Source: CAD feature listing. Evaluate the final solid. Frame: model axes, mm. Face numbers are marked on the shaded views. A direction names the side the tool comes from. Give positions to 0.01 mm unless a question says otherwise; leave off trailing zeros. Order: outer loops, then holes, each group sorted by start corner. A loop starts at its lowest first (then second) coordinate and runs counter-clockwise, first axis right, second up. Notation, with made-up numbers: M 43,-26.5 L 87,-26.5 A20 cw 87,-11.5 Z; hole C -5.5,-10 d6. An arc over 180 degrees is marked long. Return JSON: item names as keys, results as strings.
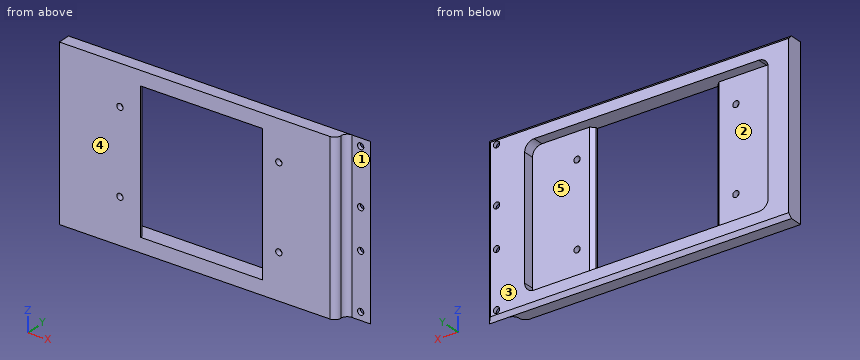
from build123d import *

# Parameters (mm, degrees)
SKETCH1_W                        = 240
SKETCH1_H                        = 133.2
BOSS_EXTRUDE1_DEPTH              = 13
CUT_EXTRUDE1_DEPTH               = 8.5
F_1_8_27_NPSM_TAPPED_HOLE1_D     = 5
F_1_8_27_NPSM_TAPPED_HOLE1_DEPTH = 22.99
F_1_8_27_NPSM_TAPPED_HOLE1_TIP   = 1.502151548
SKETCH6_W                        = 96.703687768
SKETCH6_H                        = 110.5
CUT_EXTRUDE2_DEPTH               = 144.655177421
SKETCH32_W                       = 20
SKETCH32_H                       = 133.2
CUT_EXTRUDE10_DEPTH              = 10
FILLET1_START                    = -68
FILLET1_DEPTH                    = 136
FILLET1_START_2                  = -66.6
FILLET1_2_DEPTH                  = 133.2
M6X1_0_TAPPED_HOLE1_D            = 5
M6X1_0_TAPPED_HOLE1_DEPTH        = 15
M6X1_0_TAPPED_HOLE1_TIP          = 1.502151548
CHAMFER1_SIZE                    = 3


with BuildPart() as part:
    # Sketch1 → Boss-Extrude1 (new body)
    with BuildSketch(Plane(origin=(0, 0, 0), x_dir=(1, 0, 0), z_dir=(0, 1, 0))):
        with Locations((7, 0)):
            Rectangle(SKETCH1_W, SKETCH1_H)
    extrude(amount=BOSS_EXTRUDE1_DEPTH)

    # Sketch2 → Cut-Extrude1 (cut)
    with BuildSketch(Plane(origin=(0, 13, 0), x_dir=(1, 0, 0), z_dir=(0, 1, 0))):
        with BuildLine():
            Line((-89.25, 55.25), (89.25, 55.25))
            ThreePointArc((89.25, 55.25), (94.553300859, 53.053300859), (96.75, 47.75))
            Line((96.75, 47.75), (96.75, -47.75))
            ThreePointArc((96.75, -47.75), (94.553300859, -53.053300859), (89.25, -55.25))
            Line((89.25, -55.25), (-89.25, -55.25))
            ThreePointArc((-89.25, -55.25), (-94.553300859, -53.053300859), (-96.75, -47.75))
            Line((-96.75, -47.75), (-96.75, 47.75))
            ThreePointArc((-96.75, 47.75), (-94.553300859, 53.053300859), (-89.25, 55.25))
        make_face()
    extrude(amount=-CUT_EXTRUDE1_DEPTH, mode=Mode.SUBTRACT)

    # 1/8-27 NPSM Tapped Hole1
    with Locations(Plane(origin=(0, 4.5, 0), x_dir=(1, 0, 0), z_dir=(0, 1, 0))):
        with Locations((-64.86, 30.93), (61.34, 30.93), (61.34, -34.72), (-64.86, -34.72)):
            Hole(F_1_8_27_NPSM_TAPPED_HOLE1_D / 2, depth=F_1_8_27_NPSM_TAPPED_HOLE1_DEPTH)
            with Locations((0, 0, -(F_1_8_27_NPSM_TAPPED_HOLE1_DEPTH + F_1_8_27_NPSM_TAPPED_HOLE1_TIP / 2))):  # 118° drill point
                Cone(0, F_1_8_27_NPSM_TAPPED_HOLE1_D / 2, F_1_8_27_NPSM_TAPPED_HOLE1_TIP, mode=Mode.SUBTRACT)

    # Sketch6 → Cut-Extrude2 (cut, through all)
    with BuildSketch(Plane(origin=(0, 4.5, 0), x_dir=(1, 0, 0), z_dir=(0, 1, 0))):
        Rectangle(SKETCH6_W, SKETCH6_H)
    extrude(amount=-CUT_EXTRUDE2_DEPTH, mode=Mode.SUBTRACT)

    # Sketch32 → Cut-Extrude10 (cut)
    with BuildSketch(Plane.XZ):
        with Locations((117, 0)):
            Rectangle(SKETCH32_W, SKETCH32_H)
    extrude(amount=-CUT_EXTRUDE10_DEPTH, mode=Mode.SUBTRACT)

    # Fillet1: read off the stored shape, not the designer's step
    # Fillet1 outline → Fillet1 (cut)
    with BuildSketch(Plane.XY.offset(FILLET1_START)):
        with BuildLine():
            Line((107, 0), (107, 5))
            ThreePointArc((107, 5), (105.535533906, 1.464466094), (102, 0))
            Line((102, 0), (107, 0))
        make_face()
    extrude(amount=FILLET1_DEPTH, mode=Mode.SUBTRACT)

    # Fillet1 2 outline → Fillet1 2 (add)
    with BuildSketch(Plane.XY.offset(FILLET1_START_2)):
        with BuildLine():
            ThreePointArc((107, 5), (108.464466094, 8.535533906), (112, 10))
            Line((112, 10), (107, 10))
            Line((107, 10), (107, 5))
        make_face()
    extrude(amount=FILLET1_2_DEPTH)

    # M6x1.0 Tapped Hole1
    with Locations(Plane(origin=(0, 13, 0), x_dir=(1, 0, 0), z_dir=(0, 1, 0))):
        with Locations((119.05, 60.25), (119.05, 15.75), (119.05, -16.05), (119.05, -60.55)):
            Hole(M6X1_0_TAPPED_HOLE1_D / 2, depth=M6X1_0_TAPPED_HOLE1_DEPTH)
            with Locations((0, 0, -(M6X1_0_TAPPED_HOLE1_DEPTH + M6X1_0_TAPPED_HOLE1_TIP / 2))):  # 118° drill point
                Cone(0, M6X1_0_TAPPED_HOLE1_D / 2, M6X1_0_TAPPED_HOLE1_TIP, mode=Mode.SUBTRACT)

    # Chamfer1
    chamfer1_edges = [part.edges().sort_by_distance(p)[0] for p in [
        (7, 13, 66.6),
        (127, 13, 0),
        (7, 13, -66.6),
        (48.351843884, 4.5, 0),
        (-48.351843884, 4.5, 0),
    ]]
    chamfer(chamfer1_edges, length=CHAMFER1_SIZE - 0.0001)  # a hair under: the kernel refuses the full size


solid = part.part
1. Section query A-A (z = 16.05). State how many separate pieces and enclosed holes the cut face has, then the cut area to 3 significant figures.
Evaluation:
{"separate pieces": "3", "enclosed holes": "0", "area": "812 mm^2"}
2. Draft query along X for the marked faces 4 and 5. Return one class per face: pulls with the +X half, pulls with the -X half, needs draft (parallel to the pull), parting line crosses it, or undercut.
Evaluation:
{"face 4": "needs draft", "face 5": "undercut"}
3. Section query C-C (x = -64.86). Return loops of the section in (y, z).
Evaluation:
{"outline": "M 0,-66.6 L 10,-66.6 L 13,-63.6 L 13,-55.25 L 4.5,-55.25 L 4.5,-33.43 L 0,-33.43 Z; M 0,-28.43 L 4.5,-28.43 L 4.5,32.22 L 0,32.22 Z; M 0,37.22 L 4.5,37.22 L 4.5,55.25 L 13,55.25 L 13,63.6 L 10,66.6 L 0,66.6 Z"}
4. First-contact query: pin 1 (8 mm diameter, centred on x = -64.86, z = 34.72, fed in from +Y); pin 2 (1.5 mm diameter, centred on y = 8, z = 15.5, fed in from +X); pin 3 (4 mm diameter, centred on y = 9.5, z = -13.5, fed in from +X). Flat tips, straight axial feed; report the tip coordinate or a pass-through.
Evaluation:
{"pin 1": "stops at y = 4.5", "pin 2": "stops at x = 108.69", "pin 3": "stops at x = 127"}
5. Ray query, probe 1 along Z at (x, y) = (61.34, 3.1); probe 2 along Z at (x, y) = (119.05, 11.7); probe 3 along Z at (x, y) = (-38.5, 10). Return the intervals inside material, ascending.
Evaluation:
{"probe 1": "z = -66.6 to -33.43, -28.43 to 32.22, 37.22 to 66.6", "probe 2": "z = -64.9 to -62.75, -57.75 to -18.25, -13.25 to 13.55, 18.55 to 58.05, 63.05 to 64.9", "probe 3": "z = -66.6 to -55.25, 55.25 to 66.6"}
6. Set-up query: the marked faces 1, 2 and 3. Return all of +Z, -Z, +X, -X, +Y, -Y with unobstructed straight access to the full face (end or side cutting, diameter ignored); none if empty.
Evaluation:
{"face 1": "+Z, -Z, +X, -Y", "face 2": "+Y", "face 3": "+Z, -Z, +X, -X, +Y"}
